The figure shows three views and two pictorial views of one solid part (mm, origin at its lowest corner). Answer the questions. A direction names the side the tool comes from. Coordinates: 2 decimals unless noted, no trailing zeros. Order: outer loops, then holes, each group sorted by start corner. A loop starts at its lowest first (then second) coordinate and runs counter-clockwise, first axis right, second up. Notation, with made-up numbers: (-19.75, -26) - (15.25, -26) arc R14 cw to (15.25, -6) - close; hole circle Ø4 at (13.5, 48.5). An arc over 180 degrees is marked (long way). Use one line per item in the form item = value.
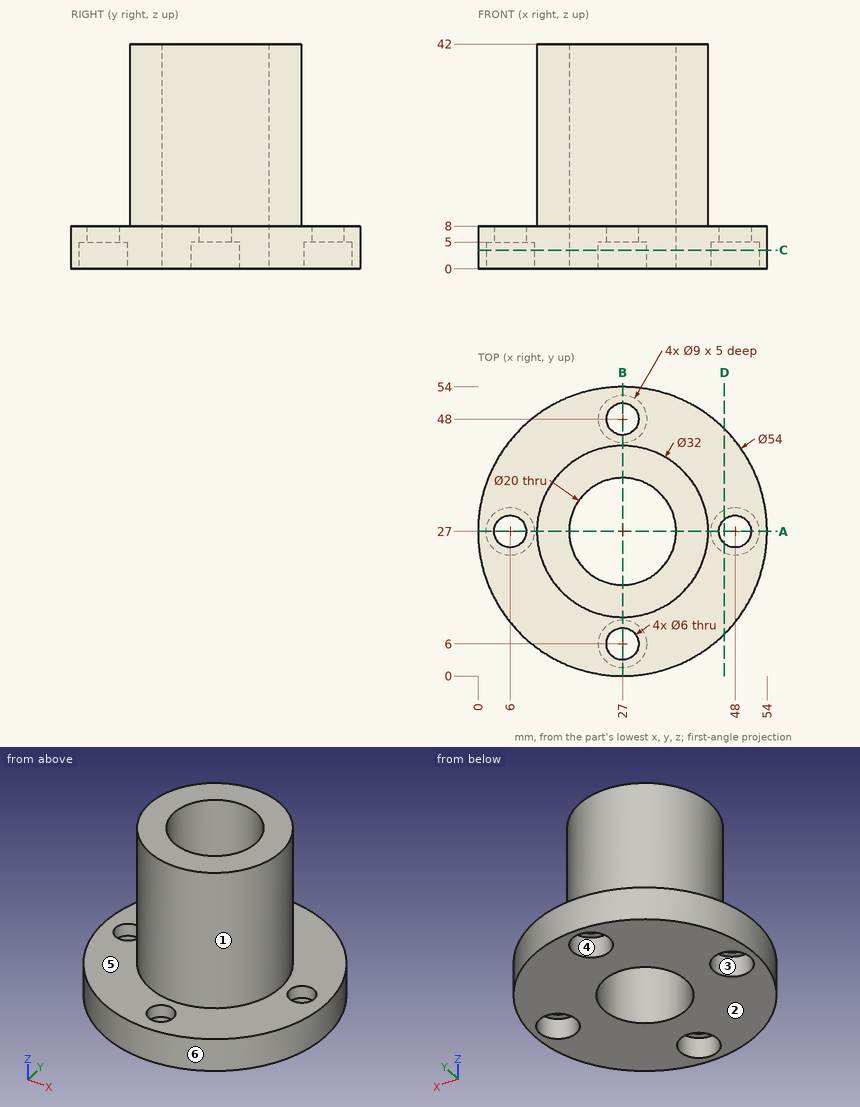
(1) Straight lines are drawn through the part: L1, parallel to Y at x = 27, z = 2; L2, parallel to Z at x = 15, y = 39.5; L3, parallel to X at y = 25, z = 20.5. For each, find the intervals that lie inside material, in ascending order.
Answer list:
L1 = 0 to 1.5, 10.5 to 17, 37 to 43.5, 52.5 to 54
L2 = 0 to 8
L3 = 11.13 to 17.2, 36.8 to 42.87
(2) Section D-D, the plane x = 46 is taken. Write down the section's boundary in (y, z), then the cut area to 3 significant figures.
Answer list:
outline = (7.82, 0) - (22.97, 0) - (22.97, 5) - (24.76, 5) - (24.76, 8) - (7.82, 8) - close; (29.24, 5) - (31.03, 5) - (31.03, 0) - (46.18, 0) - (46.18, 8) - (29.24, 8) - close
area = 253 mm2
(3) Section C-C, the plane z = 3.5 is taken. Write down the section's boundary in (x, y), then the cut area to 3 significant figures.
Answer list:
outline = circle Ø54 at (27, 27); hole circle Ø9 at (6, 27); hole circle Ø20 at (27, 27); hole circle Ø9 at (27, 6); hole circle Ø9 at (27, 48); hole circle Ø9 at (48, 27)
area = 1,720 mm2
(4) The mould has two halves that part along X. Classify the marked faces 4, 5 and 6: +X half, -X half, draft (parallel to the pull), parting line (faces both ways), or undercut.
Answer list:
face_4 = undercut
face_5 = draft
face_6 = parting line
(5) Which of the six approach directions +Z, -Z, +X, -X, +Y, -Y give full straight-line access (tool end or side, diameter ignored) to the marked faces 1, 2 and 3?
Answer list:
face_1 = +Z
face_2 = -Z, +X, -X, +Y, -Y
face_3 = -Z
(6) Given pin 1 Ø1.5 at (x, y) = (46, 41.5) entering from +Z; pin 2 Ø10 at (x, z) = (31, 14.5) entering from +Y; pin 3 Ø8 at (x, z) = (42, 16.5) entering from -Y, each flat-ended and moving along its own axis, determine where each tip first touches the part or whether it passes through.
Answer list:
pin_1 = 8
pin_2 = 43
pin_3 = 15.38
(7) Section A-A, the plane y = 27 is taken. Write down the section's boundary in (x, z).
Answer list:
outline = (0, 0) - (1.5, 0) - (1.5, 5) - (3, 5) - (3, 8) - (0, 8) - close; (9, 5) - (10.5, 5) - (10.5, 0) - (17, 0) - (17, 42) - (11, 42) - (11, 8) - (9, 8) - close; (37, 0) - (43.5, 0) - (43.5, 5) - (45, 5) - (45, 8) - (43, 8) - (43, 42) - (37, 42) - close; (51, 5) - (52.5, 5) - (52.5, 0) - (54, 0) - (54, 8) - (51, 8) - close
